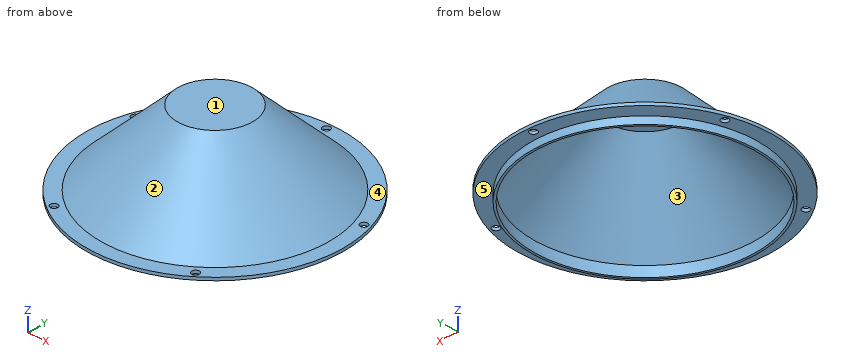
```python
from build123d import *

# Parameters (mm, degrees)
F0_R     = 171
F0_R_2   = 148
F1_DEPTH = 4
F2_R     = 5
F3_DEPTH = 4.001
F4_R     = 151
F4_R_2   = 148
F5_DEPTH = 10


with BuildPart() as f1:
    # F0 (on Top) → F1 (new body)
    with BuildSketch(Plane.XY):
        Circle(F0_R)
        Circle(F0_R_2, mode=Mode.SUBTRACT)
    extrude(amount=F1_DEPTH)

    # F2 (on face) → F3 (cut, through all)
    with BuildSketch(Plane.XY.offset(4)):
        with Locations((0, 163)):
            Circle(F2_R)
        with Locations((-155.0222121561, 50.3697700831)):
            Circle(F2_R)
        with Locations((155.0222121561, 50.3697700831)):
            Circle(F2_R)
        with Locations((95.8089961237, -131.8697700831)):
            Circle(F2_R)
        with Locations((-95.8089961237, -131.8697700831)):
            Circle(F2_R)
    extrude(amount=-F3_DEPTH, mode=Mode.SUBTRACT)

    # F4 (on face) → F5 (join)
    with BuildSketch(Plane(origin=(0, 0, 0), x_dir=(1, 0, 0), z_dir=(0, 0, -1))):
        Circle(F4_R)
        Circle(F4_R_2, mode=Mode.SUBTRACT)
    extrude(amount=F5_DEPTH)

    # F7 (on offset) → F8 (revolve)
    with BuildSketch(Plane.XZ):
        Polygon((-50, 102), (-151.8850358972, 4), (-149, 4), (-49.1942505497, 100), (0, 100), (0, 102), align=None)
    revolve(axis=Axis((0, 0, 51), (0, 0, 1)))


solid = f1.part
```
Here's how the part is built. I have some questions about the finished solid (model axes, mm). Face numbers are marked on the shaded views. A direction names the side the tool comes from. Coordinates: 2 decimals unless noted, no trailing zeros. Order: outer loops, then holes, each group sorted by start corner. A loop starts at its lowest first (then second) coordinate and runs counter-clockwise, first axis right, second up.
Item 1: If we section it at A-A, the plane x = 0: List the corners of the cut face in (y, z) for me.
Response values:
outline: (-171, 0) - (-151, 0) - (-151, -10) - (-148, -10) - (-148, 4) - (-149, 4) - (-49.19, 100) - (49.19, 100) - (149, 4) - (148, 4) - (148, -10) - (151, -10) - (151, 0) - (158, 0) - (158, 4) - (151.89, 4) - (50, 102) - (-50, 102) - (-151.89, 4) - (-171, 4) - close; (168, 0) - (171, 0) - (171, 4) - (168, 4) - close
Item 2: Which directions (+Z, -Z, +X, -X, +Y, -Y) give clear straight access to the entire face, cutting with the end or side of a thin tool? Please do the marked faces 4 and 5.
Response values:
face 4: +Z
face 5: -Z
Item 3: If we section it at C-C, the plane y = 163: List the corners of the cut face in (x, z) for me, then the cut area to 3 significant figures.
Response values:
outline: (-51.69, 0) - (-5, 0) - (-5, 4) - (-51.69, 4) - close; (5, 0) - (51.69, 0) - (51.69, 4) - (5, 4) - close
area: 374 mm2
Item 4: If we section it at D-D, the plane z = 78: List the corners of the cut face in (x, y) for me.
Response values:
outline: circle Ø149.9 at (0, 0); hole circle Ø144.13 at (0, 0)
Item 5: If we section it at B-B, the plane y = 0: List the corners of the cut face in (x, z) for me.
Response values:
outline: (-171, 0) - (-151, 0) - (-151, -10) - (-148, -10) - (-148, 4) - (-149, 4) - (-49.19, 100) - (49.19, 100) - (149, 4) - (148, 4) - (148, -10) - (151, -10) - (151, 0) - (171, 0) - (171, 4) - (151.89, 4) - (50, 102) - (-50, 102) - (-151.89, 4) - (-171, 4) - close
Item 6: I need wall thicknesses on probe 1 along Y at (x, z) = (0, 1); probe 2 along X at (y, z) = (-2.5, 93); probe 3 along Y at (x, z) = (0, -5). Which ranges of each line are inside material? Lowest first, please.
Response values:
probe 1: y = -171 to -148, 148 to 158, 168 to 171
probe 2: x = -59.3 to -56.42, 56.42 to 59.3
probe 3: y = -151 to -148, 148 to 151
Item 7: Thinking about a two-plate mould opening in Y: for the marked faces 1, 2 and 3, which applies, pulls with the +Y half, pulls with the -Y half, needs draft (parallel to the pull), parting line crosses it, or undercut?
Response values:
face 1: needs draft
face 2: parting line crosses it
face 3: undercut
Item 8: I'm going to push flat-ended pins straight in: pin 1 Ø8 at (x, y) = (-9, 31.5) entering from -Z; pin 2 Ø16 at (x, y) = (155.02, 50.37) entering from -Z; pin 3 Ø1 at (x, y) = (-94.5, 58) entering from +Z; pin 4 Ø6 at (x, y) = (-155.02, 50.37) entering from -Z. Where does each tip first touch, or does it pass through?
Response values:
pin 1: stops at z = 100
pin 2: stops at z = 0
pin 3: stops at z = 43.92
pin 4: passes through
